```python
from build123d import *

# Parameters (mm, degrees)
SKETCH1_R           = 1
SKETCH1_R_2         = 2.5
BOSS_EXTRUDE1_DEPTH = 2
SKETCH2_R           = 3.65
SKETCH2_R_2         = 2.5
BOSS_EXTRUDE2_DEPTH = 2.5


with BuildPart() as part:
    # Sketch1 → Boss-Extrude1 (new body)
    with BuildSketch(Plane(origin=(0, 0, 0), x_dir=(1, 0, 0), z_dir=(0, 1, 0))):
        with BuildLine():
            Line((3, -2.079062289), (1.993477511, -14.51139211))
            ThreePointArc((1.993477511, -14.51139211), (0, -16.35), (-1.993477511, -14.51139211))
            Line((-1.993477511, -14.51139211), (-3, -2.079062289))
            ThreePointArc((-3, -2.079062289), (0, 3.65), (3, -2.079062289))
        make_face()
        with Locations((0, -6.65)):
            Circle(SKETCH1_R, mode=Mode.SUBTRACT)
        with Locations((0, -10.65)):
            Circle(SKETCH1_R, mode=Mode.SUBTRACT)
        Circle(SKETCH1_R_2, mode=Mode.SUBTRACT)
    boss_extrude1 = extrude(amount=BOSS_EXTRUDE1_DEPTH)

    # Sketch2 → Boss-Extrude2 (add)
    with BuildSketch(Plane(origin=(0, 2, 0), x_dir=(1, 0, 0), z_dir=(0, 1, 0))):
        Circle(SKETCH2_R)
        Circle(SKETCH2_R_2, mode=Mode.SUBTRACT)
    boss_extrude2 = extrude(amount=BOSS_EXTRUDE2_DEPTH)

    # Mirror1: Boss-Extrude1, Boss-Extrude2 across plane
    add(boss_extrude1.mirror(Plane.XY))
    add(boss_extrude2.mirror(Plane.XY))


solid = part.part
```
Could you check a few things on this model? Use its own coordinates, in mm. Round coordinates to 2 decimals unless told otherwise and drop trailing zeros. Write each loop counter-clockwise with the first axis right and the second up, starting at its lowest first coordinate (ties: lowest second). Pieces come first, ordered by that corner, then holes. Notation, with made-up numbers: M 17.25,-12.75 L 30.25,-12.75 A31 ccw 30.25,24.25 Z; hole C 49.25,11 d1. An arc over 180 degrees is marked long. Answer in a Markdown table with one row per item. Add a question column.
Q1. Imagine slicing it at D-D (x = -1.5). Please give me the cut outline in (y, z).
Q2. If we mould it in two halves opening along Z, with no side actions, what happens to faces 1 (the cylindrical face through (-0.13, 0.99, -5.66)), 2 (the flat face through (2.504, 0.986, -8.208)), 3 (the flat face through (0, 2, 9))? For each: +Z half, -Z half, draft (parallel to the pull), parting line (faces both ways), or undercut.
Q3. Imagine slicing it at B-B (y = 0.35). Please give me the cut outline in (x, z), then the cut area to 3 significant figures.
Q4. Imagine slicing it at C-C (x = 0). Please give me the cut outline in (y, z).
Q5. Will these pins go through, and if not, where does the flat tip stop? pin 1 Ø2 at (y, z) = (3.5, -3.5) entering from +X; pin 2 Ø1.8 at (x, z) = (0.5, -12.5) entering from +Y; pin 3 Ø1 at (y, z) = (1.5, 7.5) entering from -X.
Q6. If I drill on line 1 (X direction, y = 3.2, z = 0); line 2 (Y direction, x = -1.5, z = 7.5); line 3 (Z direction, x = -1.25, y = 3.2), over which ranges is the centre line in solid material (lowest first)? Write a range as from..to.
Q7. Imagine slicing it at A-A (z = 0). Please give me the cut outline in (x, y), then the cut area to 4 significant figures.
Values:
| question | item | result |
|---|---|---|
| 1 | outline | M 0,-15.67 L 2,-15.67 L 2,-3.33 L 4.5,-3.33 L 4.5,-2 L 0,-2 Z; M 0,2 L 4.5,2 L 4.5,3.33 L 2,3.33 L 2,15.67 L 0,15.67 Z |
| 2 | face 1 | undercut |
| 2 | face 2 | -Z half |
| 2 | face 3 | draft |
| 3 | outline | M -3,-2.08 L -1.99,-14.51 A2 ccw 1.99,-14.51 L 3,-2.08 A3.65 ccw 3,2.08 L 1.99,14.51 A2 ccw -1.99,14.51 L -3,2.08 A3.65 ccw Z; hole C 0,0 d5; hole C 0,-10.65 d2; hole C 0,-6.65 d2; hole C 0,6.65 d2; hole C 0,10.65 d2 |
| 3 | area | 132 mm^2 |
| 4 | outline | M 0,-16.35 L 2,-16.35 L 2,-11.65 L 0,-11.65 Z; M 0,-9.65 L 2,-9.65 L 2,-7.65 L 0,-7.65 Z; M 0,-5.65 L 2,-5.65 L 2,-3.65 L 4.5,-3.65 L 4.5,-2.5 L 0,-2.5 Z; M 0,2.5 L 4.5,2.5 L 4.5,3.65 L 2,3.65 L 2,5.65 L 0,5.65 Z; M 0,7.65 L 2,7.65 L 2,9.65 L 0,9.65 Z; M 0,11.65 L 2,11.65 L 2,16.35 L 0,16.35 Z |
| 5 | pin 1 | x = 2.66 |
| 5 | pin 2 | y = 2 |
| 5 | pin 3 | x = -2.6 |
| 6 | line 1 | -3.65..-2.5, 2.5..3.65 |
| 6 | line 2 | 0..2 |
| 6 | line 3 | -3.43..-2.17, 2.17..3.43 |
| 7 | outline | M -3.65,0 L -2.5,0 L -2.5,4.5 L -3.65,4.5 Z; M 2.5,0 L 3.65,0 L 3.65,4.5 L 2.5,4.5 Z |
| 7 | area | 10.35 mm^2 |
